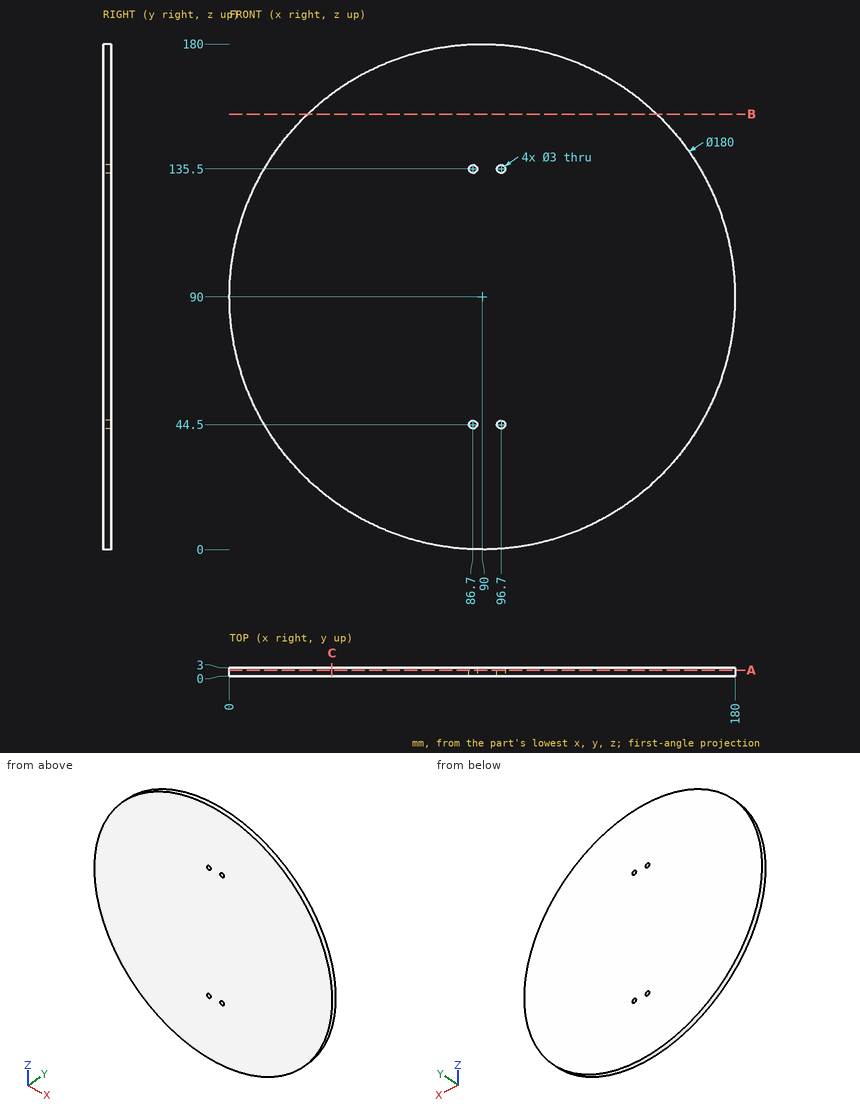
Source: three-view drawing plus pictorial views. Frame: mm from the lowest corner of the part. Give positions to 0.01 mm unless a question says otherwise; leave off trailing zeros. Order: outer loops, then holes, each group sorted by start corner. A loop starts at its lowest first (then second) coordinate and runs counter-clockwise, first axis right, second up.
1. Section A-A on y = 2.1. Return the cut outline in (x, z), and give its area (3 significant figures).
Derived:
outline: circle Ø180 at (90, 90); hole circle Ø3 at (86.7, 44.5); hole circle Ø3 at (86.7, 135.5); hole circle Ø3 at (96.7, 44.5); hole circle Ø3 at (96.7, 135.5)
area: 25,400 mm2
2. Material intervals for L1, parallel to Z at x = 86.7, y = 1.35; L2, parallel to Z at x = 96.7, y = 1.4; L3, parallel to X at y = 2.05, z = 135.5, sorted ascending.
Derived:
L1: z = 0.06 to 43, 46 to 134, 137 to 179.94
L2: z = 0.25 to 43, 46 to 134, 137 to 179.75
L3: x = 12.35 to 85.2, 88.2 to 95.2, 98.2 to 167.65
3. Section B-B on z = 155. Return the cut outline in (x, y), and give its area (3 significant figures).
Derived:
outline: (27.75, 0) - (152.25, 0) - (152.25, 3) - (27.75, 3) - close
area: 373 mm2
4. Section C-C on x = 36.5. Return the cut outline in (y, z).
Derived:
outline: (0, 17.63) - (3, 17.63) - (3, 162.37) - (0, 162.37) - close
5. Pin query (flat end, axial travel): pin 1 (6 mm diameter, centred on x = 148, z = 69.5, fed in from -Y); pin 2 (1.5 mm diameter, centred on y = 1, z = 146.5, fed in from +X); pin 3 (1.5 mm diameter, centred on y = 2, z = 152, fed in from +X). Return the tip coordinate at first contact, or that it passes through.
Derived:
pin 1: stops at y = 0
pin 2: stops at x = 160.65
pin 3: stops at x = 155.94
